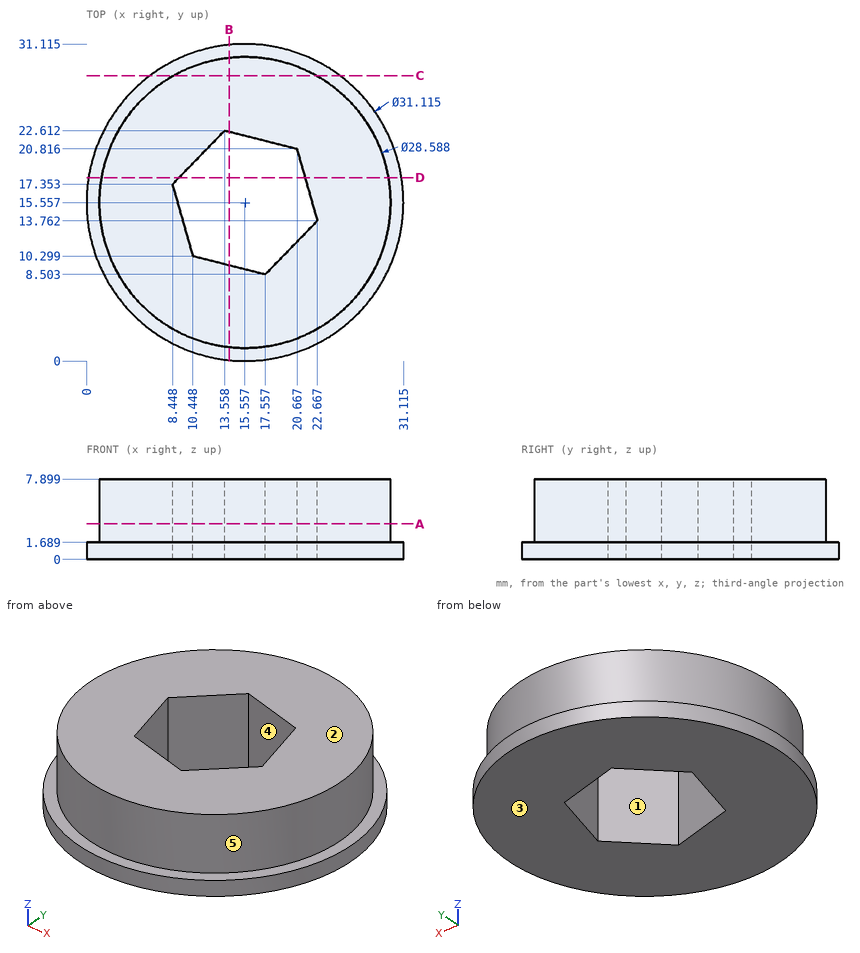
For this review, use the dimensioned drawing (mm, ordinates from the lowest corner) and the shaded views. A direction names the side the tool comes from. Coordinates: 2 decimals unless noted, no trailing zeros. Write each loop counter-clockwise with the first axis right and the second up, starting at its lowest first coordinate (ties: lowest second). Pieces come first, ordered by that corner, then holes. Notation, with made-up numbers: (12, 5.5) - (19, 5.5) arc R31 cw to (19, 39.5) - close; hole circle Ø5 at (40, 65.5). An arc over 180 degrees is marked (long way). Answer in a Markdown table with one row per item. Add a question column.
Q1. To check wall thickness, follow line 1 along X through (y, z) = (12, 3.75) (1 decimal); line 2 along Y through (x, z) = (17.5, 2.75) (1 decimal); line 3 along X through (y, z) = (14.5, 6). State the ranges of each line that lie inside material, in increasing order. Write a range as from..to.
Q2. Consider section D-D on y = 18. Give the boundary of the cut face in (x, z) (1 decimal), then the cut area to 3 significant figures.
Q3. Consider section B-B on x = 14. Give the boundary of the cut face in (y, z).
Q4. Consider section A-A on z = 3.5. Give the boundary of the cut face in (x, y), then the cut area to 3 significant figures.
Q5. Clearance check with flat-ended pins moving along their axes: pin 1 (2 mm diameter, centred on x = 13, z = 5.5, fed in from -Y); pin 2 (2 mm diameter, centred on y = 7.5, z = 4.5, fed in from +X); pin 3 (1 mm diameter, centred on x = 22.5, z = 5.5, fed in from -Y). State where each tip first meets the part, or that it passes through.
Q6. Consider section C-C on y = 28. Give the boundary of the cut face in (x, z).
Q7. Draft analysis for pull direction Z (two halves, no side actions). For the marked faces 1, 2 and 3, state which applies: +Z half, -Z half, draft (parallel to the pull), parting line (faces both ways), or undercut.
Q8. For the marked faces 4 and 5, list the 3-axis set-ups (+Z, -Z, +X, -X, +Y, -Y) from which the entire face can be reached by the end or side of a thin tool; tool diameter is ignored.
Answers below:
| question | item | result |
|---|---|---|
| 1 | line 1 | 1.7..10, 21..29.4 |
| 1 | line 2 | 1.4..8.5, 21.6..29.7 |
| 1 | line 3 | 1.3..9.26, 22.46..29.81 |
| 2 | outline | (0.2, 0) - (9.1, 0) - (9.1, 7.9) - (1.5, 7.9) - (1.5, 1.7) - (0.2, 1.7) - close; (21.5, 0) - (30.9, 0) - (30.9, 1.7) - (29.6, 1.7) - (29.6, 7.9) - (21.5, 7.9) - close |
| 2 | area | 129 mm² |
| 3 | outline | (0.08, 0) - (9.4, 0) - (9.4, 7.9) - (1.35, 7.9) - (1.35, 1.69) - (0.08, 1.69) - close; (22.5, 0) - (31.04, 0) - (31.04, 1.69) - (29.77, 1.69) - (29.77, 7.9) - (22.5, 7.9) - close |
| 4 | outline | circle Ø28.59 at (15.56, 15.56); hole (8.45, 17.35) - (10.45, 10.3) - (17.56, 8.5) - (22.67, 13.76) - (20.67, 20.82) - (13.56, 22.61) - close |
| 4 | area | 502 mm² |
| 5 | pin 1 | y = 1.35 |
| 5 | pin 2 | x = 27.99 |
| 5 | pin 3 | y = 2.8 |
| 6 | outline | (6.22, 0) - (24.9, 0) - (24.9, 1.69) - (22.59, 1.69) - (22.59, 7.9) - (8.52, 7.9) - (8.52, 1.69) - (6.22, 1.69) - close |
| 7 | face 1 | draft |
| 7 | face 2 | +Z half |
| 7 | face 3 | -Z half |
| 8 | face 4 | +Z, -Z |
| 8 | face 5 | +Z |
